Could you check a few things on this model? Use its own coordinates, in mm. Face numbers are marked on the shaded views. A direction names the side the tool comes from. Give positions to 0.01 mm unless a question says otherwise; leave off trailing zeros. Write each loop counter-clockwise with the first axis right and the second up, starting at its lowest first coordinate (ties: lowest second). Pieces come first, ordered by that corner, then holes. Notation, with made-up numbers: (67.5, 38) - (89.5, 38) arc R25 cw to (89.5, 77) - close; hole circle Ø2 at (4.5, -16.5). An arc over 180 degrees is marked (long way). Answer as CSV lines item,"result". Start each with the question number.
Q1. Imagine slicing it at A-A on y = 34.5. List the corners of the cut face in (x, z) for me.
Q2. If I drill on line 1 along Y through (x, z) = (-12.9, 0); line 2 along Z through (x, y) = (12.75, 13); line 3 along X through (y, z) = (68.5, -4.5), over which ranges is the centre line in solid material (lowest first)?
Q3. We'd pull the mould along X, two halves only. Please class the marked faces 4, 5 and 6: pulls with the +X half, pulls with the -X half, needs draft (parallel to the pull), parting line crosses it, or undercut.
Q4. Imagine slicing it at D-D on z = 4.75. List the corners of the cut face in (x, y) for me, and give its area (3 significant figures).
Q5. Will these pins go through, and if not, where does the flat tip stop? pin 1 Ø7 at (x, z) = (0, 0) entering from +Y; pin 2 Ø4.5 at (y, z) = (67, 0) entering from -X.
Q6. Imagine slicing it at B-B on y = 43.5. List the corners of the cut face in (x, z) for me.
Q7. On a 3-axis mill with a long thin cutter (end or side, diameter ignored), from which of +Z, -Z, +X, -X, +Y, -Y can I reach the whole of each face in a straight line? I mean the marked faces 1, 2 and 3. Say none if no direction works.
Q8. Imagine slicing it at C-C on x = 0. List the corners of the cut face in (y, z) for me, and give its area (3 significant figures).
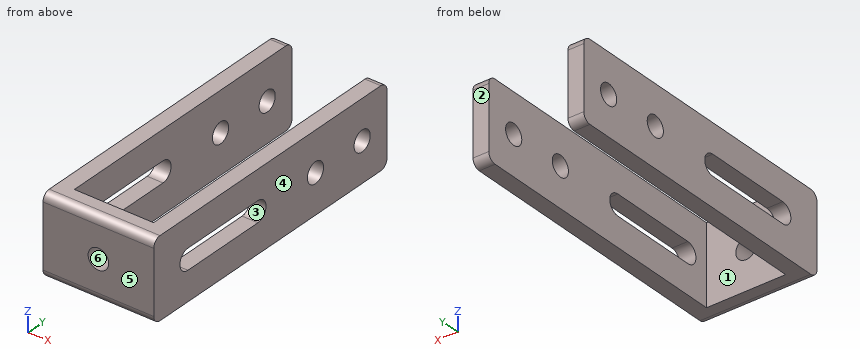
```python
from build123d import *

# Parameters (mm, degrees)
SKETCH1_W           = 28
SKETCH1_H           = 20
BOSS_EXTRUDE1_DEPTH = 5
SKETCH2_W           = 4
SKETCH2_H           = 20
BOSS_EXTRUDE2_DEPTH = 70
SKETCH3_R           = 2.6
CUT_EXTRUDE1_DEPTH  = 5
SKETCH4_R           = 2.6
CUT_EXTRUDE2_DEPTH  = 40
FILLET1_R           = 2


with BuildPart() as part:
    # Sketch1 → Boss-Extrude1 (new body)
    with BuildSketch(Plane(origin=(0, 0, 0), x_dir=(1, 0, 0), z_dir=(0, 1, 0))):
        Rectangle(SKETCH1_W, SKETCH1_H)
    extrude(amount=BOSS_EXTRUDE1_DEPTH)

    # Sketch2 → Boss-Extrude2 (add)
    with BuildSketch(Plane(origin=(0, 5, 0), x_dir=(1, 0, 0), z_dir=(0, 1, 0))):
        with Locations((-12, 0)):
            Rectangle(SKETCH2_W, SKETCH2_H)
        with Locations((12, 0)):
            Rectangle(SKETCH2_W, SKETCH2_H)
    extrude(amount=BOSS_EXTRUDE2_DEPTH)

    # Sketch3 → Cut-Extrude1 (cut)
    with BuildSketch(Plane.XZ):
        with Locations(Location((0, 0, 0), (0, 0, 270))):
            Circle(SKETCH3_R)
    extrude(amount=-CUT_EXTRUDE1_DEPTH, mode=Mode.SUBTRACT)

    # Sketch4 → Cut-Extrude2 (cut)
    with BuildSketch(Plane(origin=(14, 0, 0), x_dir=(0, 0, -1), z_dir=(1, 0, 0))):
        with Locations((0, 67)):
            Circle(SKETCH4_R)
        with Locations((0, 52)):
            Circle(SKETCH4_R)
        with BuildLine():
            Line((2.6, 33.5), (2.6, 11))
            ThreePointArc((2.6, 11), (0, 8.4), (-2.6, 11))
            Line((-2.6, 11), (-2.6, 33.5))
            ThreePointArc((-2.6, 33.5), (0, 36.1), (2.6, 33.5))
        make_face()
    extrude(amount=-CUT_EXTRUDE2_DEPTH, mode=Mode.SUBTRACT)

    # Fillet1
    fillet1_edges = [part.edges().sort_by_distance(p)[0] for p in [
        (-12, 75, 10),
        (-12, 75, -10),
        (12, 75, -10),
        (12, 75, 10),
        (0, 0, 10),
        (0, 0, -10),
    ]]
    fillet(fillet1_edges, radius=FILLET1_R)


solid = part.part
```
Conclusion:
1,outline,"(-14, -10) - (-10, -10) - (-10, -2.4) - (-14, -2.4) - close; (-14, 2.4) - (-10, 2.4) - (-10, 10) - (-14, 10) - close; (10, -10) - (14, -10) - (14, -2.4) - (10, -2.4) - close; (10, 2.4) - (14, 2.4) - (14, 10) - (10, 10) - close"
2,line 1,"0 to 8.4, 36.1 to 49.4, 54.6 to 64.4, 69.6 to 75"
2,line 2,"-10 to -2.6, 2.6 to 10"
2,line 3,"-14 to -10, 10 to 14"
3,face 4,"pulls with the +X half"
3,face 5,"needs draft"
3,face 6,"undercut"
4,outline,"(-14, 0) - (14, 0) - (14, 75) - (10, 75) - (10, 5) - (-10, 5) - (-10, 75) - (-14, 75) - close"
4,area,"700 mm^2"
5,pin 1,"y = 5"
5,pin 2,"through"
6,outline,"(-14, -10) - (-10, -10) - (-10, 10) - (-14, 10) - close; (10, -10) - (14, -10) - (14, 10) - (10, 10) - close"
7,face 1,"+Z, -Z, +Y"
7,face 2,"+Z, -Z, +X, -X, +Y"
7,face 3,"+X, -X"
8,outline,"(0, -8) arc R2 ccw to (2, -10) - (5, -10) - (5, -2.6) - (0, -2.6) - close; (0, 2.6) - (5, 2.6) - (5, 10) - (2, 10) arc R2 ccw to (0, 8) - close"
8,area,"72.3 mm^2"
